Verification items for the finished model (mm, model axes). A direction names the side the tool comes from. Give positions to 0.01 mm unless a question says otherwise; leave off trailing zeros. Order: outer loops, then holes, each group sorted by start corner. A loop starts at its lowest first (then second) coordinate and runs counter-clockwise, first axis right, second up. Notation, with made-up numbers: (15.25, -33) -> (24.25, -33) arc R18 cw to (24.25, -7) -> close; hole circle Ø10 at (-8, -19.75). An arc over 180 degrees is marked (long way). One line per question, with ' | ' between items. Start each with the question number.
Q1. Section check D-D on x = 11.5. Record the cut outline in (y, z).
Q2. Go/stop test with flat-tipped pins: pin 1 (1.2 mm diameter, centred on y = 1, z = 2, fed in from +X); pin 2 (1 mm diameter, centred on x = 6, y = 2, fed in from +Z). Record where each tip stops, or that it passes through.
Q3. Material ranges on probe 1 along Z at (x, y) = (-2.5, 2.1); probe 2 along X at (y, z) = (2.3, -1); probe 3 along X at (y, z) = (2.3, 5.25), recorded low to high. Write a range as [from, to].
Q4. Section check B-B on x = -1.25. Record the cut outline in (y, z).
Q5. Access from +Z, -Z, +X, -X, +Y, -Y to the whole of each face (thin tool, end or side, straight path). Record for faces 5 (the flat face through (14, 2, 0)), 6 (the flat face through (6.5, 2, 0)).
Q6. Section check A-A on z = -5. Record the cut outline in (x, y), plus the area to 3 significant figures.
Q7. Section check C-C on y = 3.25. Record the cut outline in (x, z).
Q8. Mould release check, pull along X, two halves, no side actions. Record for faces 1 (the flat face through (0, 2, -10)), 2 (the cylindrical face through (-6.87, 1.97, -9.61)), 3 (the cylindrical face through (13.61, 1.97, -2.87)), 4 (the flat face through (0, 2, 7.25)): released by +X, released by -X, zero draft, split by the parting line, or undercut.
from build123d import *

# Parameters (mm, degrees)
ESQUISSE1_W             = 28
ESQUISSE1_H             = 20
BOSS_EXTRU_1_DEPTH      = 4
ESQUISSE2_W             = 13
ESQUISSE2_H             = 14.5
ENL_V_MAT_EXTRU_1_DEPTH = 4
ENL_V_MAT_EXTRU_2_DEPTH = 4
CONG_2_R                = 5


with BuildPart() as part:
    # Esquisse1 → Boss.-Extru.1 (new body)
    with BuildSketch(Plane(origin=(0, 0, 0), x_dir=(1, 0, 0), z_dir=(0, 1, 0))):
        Rectangle(ESQUISSE1_W, ESQUISSE1_H)
    extrude(amount=BOSS_EXTRU_1_DEPTH)

    # Esquisse2 → Enlèv. mat.-Extru.1 (cut)
    with BuildSketch(Plane(origin=(0, 4, 0), x_dir=(1, 0, 0), z_dir=(0, 1, 0))):
        Rectangle(ESQUISSE2_W, ESQUISSE2_H)
    extrude(amount=-ENL_V_MAT_EXTRU_1_DEPTH, mode=Mode.SUBTRACT)

    # Esquisse3 → Enlèv. mat.-Extru.2 (cut)
    with BuildSketch(Plane(origin=(0, 4, 0), x_dir=(1, 0, 0), z_dir=(0, 1, 0))):
        Polygon((-14, 10), (-14, 3), (-7, 10), align=None)
        Polygon((14, 10), (7, 10), (14, 3), align=None)
        Polygon((14, -3), (7, -10), (14, -10), align=None)
        Polygon((-7, -10), (-14, -3), (-14, -10), align=None)
    extrude(amount=-ENL_V_MAT_EXTRU_2_DEPTH, mode=Mode.SUBTRACT)

    # Congé2
    cong_2_edges = [part.edges().sort_by_distance(p)[0] for p in [
        (-14, 2, 3),
        (-7, 2, 10),
        (7, 2, 10),
        (14, 2, 3),
        (14, 2, -3),
        (7, 2, -10),
        (-14, 2, -3),
        (-7, 2, -10),
    ]]
    fillet(cong_2_edges, radius=CONG_2_R)


solid = part.part
Filled in:
1) outline: (0, -5.5) -> (4, -5.5) -> (4, 5.5) -> (0, 5.5) -> close
2) pin 1: x = 13.98 | pin 2: z = 9.97
3) probe 1: [-10, -7.25], [7.25, 10] | probe 2: [-14, -6.5], [6.5, 14] | probe 3: [-11.75, -6.5], [6.5, 11.75]
4) outline: (0, -10) -> (4, -10) -> (4, -7.25) -> (0, -7.25) -> close; (0, 7.25) -> (4, 7.25) -> (4, 10) -> (0, 10) -> close
5) face 5: +Z, -Z, +X, +Y, -Y | face 6: +Y, -Y
6) outline: (-12, 0) -> (-6.5, 0) -> (-6.5, 4) -> (-12, 4) -> close; (6.5, 0) -> (12, 0) -> (12, 4) -> (6.5, 4) -> close | area: 44.0 mm²
7) outline: (-14, -0.93) arc R5 ccw to (-12.54, -4.46) -> (-8.46, -8.54) arc R5 ccw to (-4.93, -10) -> (4.93, -10) arc R5 ccw to (8.46, -8.54) -> (12.54, -4.46) arc R5 ccw to (14, -0.93) -> (14, 0.93) arc R5 ccw to (12.54, 4.46) -> (8.46, 8.54) arc R5 ccw to (4.93, 10) -> (-4.93, 10) arc R5 ccw to (-8.46, 8.54) -> (-12.54, 4.46) arc R5 ccw to (-14, 0.93) -> close; hole (-6.5, -7.25) -> (6.5, -7.25) -> (6.5, 7.25) -> (-6.5, 7.25) -> close
8) face 1: zero draft | face 2: released by -X | face 3: released by +X | face 4: undercut
